from build123d import *

# Parameters (mm, degrees)
SKETCH1_W           = 160
SKETCH1_H           = 25
SKETCH1_R           = 6.25
BOSS_EXTRUDE1_DEPTH = 4


with BuildPart() as part:
    # Sketch1 → Boss-Extrude1 (new body)
    with BuildSketch(Plane(origin=(0, 0, 0), x_dir=(1, 0, 0), z_dir=(0, 1, 0))):
        Rectangle(SKETCH1_W, SKETCH1_H)
        with Locations((67.5, 0)):
            Circle(SKETCH1_R, mode=Mode.SUBTRACT)
    extrude(amount=BOSS_EXTRUDE1_DEPTH)


solid = part.part
The model under review builds one solid part; all positions refer to its coordinate system, in mm. Round coordinates to 2 decimals unless told otherwise and drop trailing zeros. Order: outer loops, then holes, each group sorted by start corner. A loop starts at its lowest first (then second) coordinate and runs counter-clockwise, first axis right, second up. Notation, with made-up numbers: (48, 28.25) -> (80, 28.25) arc R32 ccw to (80, 66.25) -> close; hole circle Ø11 at (15.25, 10.5). An arc over 180 degrees is marked (long way). Use CSV: the item, a comma, the result in double quotes. Start each with the question number.
(1) Insertion check: pin 1 (8 mm diameter, centred on x = 19, z = 3, fed in from -Y). The pin has a flat end and moves straight along its axis. Give the tip position at first contact, or say it passes through.
(2) Consider section A-A on z = 0. Write out the cut boundary in (x, y).
(3) Wall thickness on probe 1 along X at (y, z) = (2.7, 0); probe 2 along Z at (x, y) = (67.5, 2.1); probe 3 along X at (y, z) = (0.95, 4): over which ranges is each line inside the solid? List them lowest first. Write a range as from..to.
(4) Consider section C-C on y = 1.4. Write out the cut boundary in (x, z).
(5) Consider section B-B on x = 67.5. Write out the cut boundary in (y, z), and give its area (3 significant figures).
(6) Mouldability with a two-part tool opening along Z and no side actions: class faces 1 (the face through (73.46, 1.97, -1.88)), 2 (the face through (-1, 0, 0)), 3 (the face through (-1, 2, 12.5)) as pulls with the +Z half, pulls with the -Z half, needs draft (parallel to the pull), parting line crosses it, or undercut.
Responses:
1,pin 1,"y = 0"
2,outline,"(-80, 0) -> (61.25, 0) -> (61.25, 4) -> (-80, 4) -> close; (73.75, 0) -> (80, 0) -> (80, 4) -> (73.75, 4) -> close"
3,probe 1,"-80..61.25, 73.75..80"
3,probe 2,"-12.5..-6.25, 6.25..12.5"
3,probe 3,"-80..62.7, 72.3..80"
4,outline,"(-80, -12.5) -> (80, -12.5) -> (80, 12.5) -> (-80, 12.5) -> close; hole circle Ø12.5 at (67.5, 0)"
5,outline,"(0, -12.5) -> (4, -12.5) -> (4, -6.25) -> (0, -6.25) -> close; (0, 6.25) -> (4, 6.25) -> (4, 12.5) -> (0, 12.5) -> close"
5,area,"50.0 mm²"
6,face 1,"undercut"
6,face 2,"needs draft"
6,face 3,"pulls with the +Z half"
